Design review of the part shown in the three views and the two pictorial views. Dimensions are in mm from the part's minimum x, y and z. Round coordinates to 2 decimals unless told otherwise and drop trailing zeros. Loops run counter-clockwise (first coordinate to the right, second up) from the corner with the lowest first, then second, coordinate; pieces in that order, holes last. Notation, with made-up numbers: M 88.25,89.25 L 135.25,89.25 A26 ccw 135.25,125.25 Z; hole C 63,68.25 d2. An arc over 180 degrees is marked long. Answer as CSV lines item,"result". Start each with the question number.
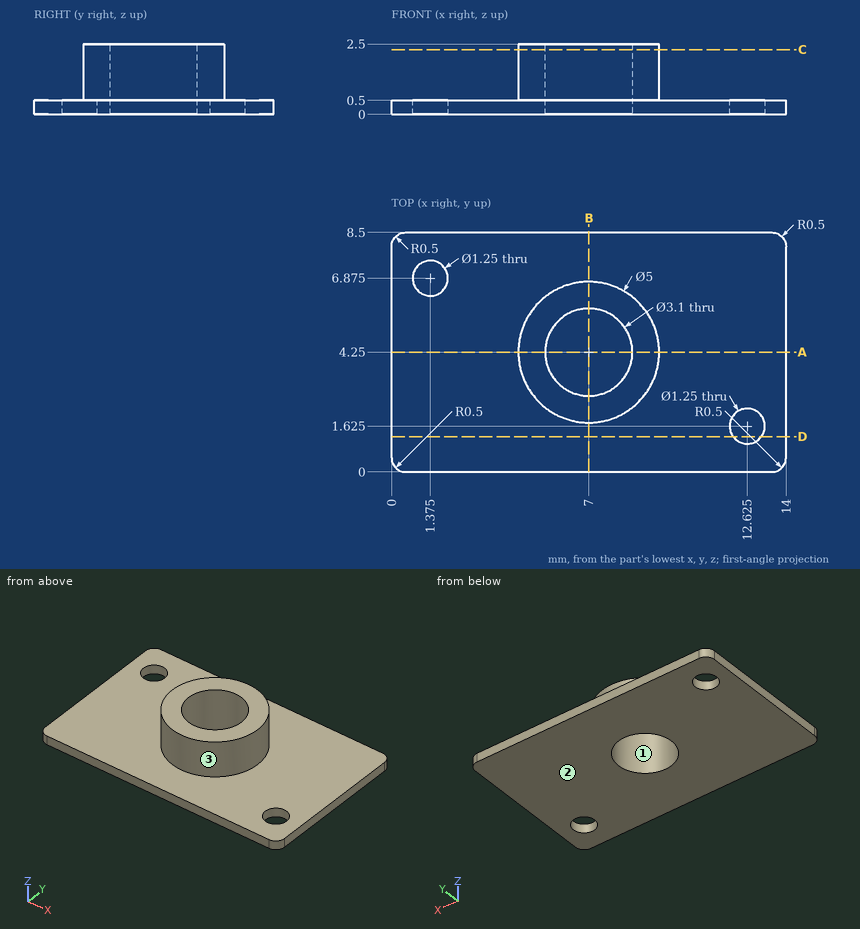
Item 1: To check wall thickness, follow line 1 (Y direction, x = 7, z = 1.65); line 2 (Z direction, x = 1.25, y = 8); line 3 (X direction, y = 4, z = 2.2). State the ranges of each line that lie inside material, in increasing order.
Item 2: Consider section A-A, the plane y = 4.25. Write out the cut boundary in (x, z), then the cut area to 3 significant figures.
Item 3: Consider section B-B, the plane x = 7. Write out the cut boundary in (y, z), then the cut area to 3 significant figures.
Item 4: Insertion check: pin 1 Ø1 at (x, y) = (1.375, 6.875) entering from -Z; pin 2 Ø2 at (x, y) = (11, 2.5) entering from +Z. Each pin has a flat end and moves straight along its axis. Give the tip position at first contact, or say it passes through.
Item 5: Consider section D-D, the plane y = 1.25. Write out the cut boundary in (x, z) (3 decimals).
Item 6: Consider section C-C, the plane z = 2.3. Write out the cut boundary in (x, y).
Item 7: The part is to be moulded in two halves that separate along X. For the marked faces 1, 2 and 3, say which applies: +X half, -X half, draft (parallel to the pull), parting line (faces both ways), or undercut.
Found:
1,line 1,"y = 1.75 to 2.7, 5.8 to 6.75"
1,line 2,"z = 0 to 0.5"
1,line 3,"x = 4.51 to 5.47, 8.53 to 9.49"
2,outline,"M 0,0 L 5.45,0 L 5.45,2.5 L 4.5,2.5 L 4.5,0.5 L 0,0.5 Z; M 8.55,0 L 14,0 L 14,0.5 L 9.5,0.5 L 9.5,2.5 L 8.55,2.5 Z"
2,area,"9.25 mm^2"
3,outline,"M 0,0 L 2.7,0 L 2.7,2.5 L 1.75,2.5 L 1.75,0.5 L 0,0.5 Z; M 5.8,0 L 8.5,0 L 8.5,0.5 L 6.75,0.5 L 6.75,2.5 L 5.8,2.5 Z"
3,area,"6.50 mm^2"
4,pin 1,"passes through"
4,pin 2,"stops at z = 0.5"
5,outline,"M 0,0 L 12.125,0 L 12.125,0.5 L 0,0.5 Z; M 13.125,0 L 14,0 L 14,0.5 L 13.125,0.5 Z"
6,outline,"C 7,4.25 d5; hole C 7,4.25 d3.1"
7,face 1,"undercut"
7,face 2,"draft"
7,face 3,"parting line"
